from build123d import *

# Parameters (mm, degrees)
SKETCH1_R           = 19
BOSS_EXTRUDE1_DEPTH = 57
SKETCH3_W           = 38
SKETCH3_H           = 38
BOSS_EXTRUDE3_DEPTH = 48
SKETCH4_R           = 6.5
BOSS_EXTRUDE4_DEPTH = 26
SKETCH5_R           = 1.5
BOSS_EXTRUDE5_DEPTH = 13
FILLET1_R           = 5
SKETCH6_R           = 2
CUT_EXTRUDE1_DEPTH  = 10
CUT_EXTRUDE2_START  = -10
SKETCH7_R           = 2
CUT_EXTRUDE2_DEPTH  = 10


with BuildPart() as part:
    # Sketch1 → Boss-Extrude1 (new body)
    with BuildSketch(Plane.XY):
        with Locations(Location((0, 0, 0), (0, 0, 180))):
            Circle(SKETCH1_R)
    extrude(amount=BOSS_EXTRUDE1_DEPTH)

    # Sketch3 → Boss-Extrude3 (add)
    with BuildSketch(Plane(origin=(0, 0, 0), x_dir=(-1, 0, 0), z_dir=(0, 0, -1))):
        Rectangle(SKETCH3_W, SKETCH3_H)
    extrude(amount=BOSS_EXTRUDE3_DEPTH)

    # Sketch4 → Boss-Extrude4 (add)
    with BuildSketch(Plane(origin=(0, 0, -48), x_dir=(-1, 0, 0), z_dir=(0, 0, -1))):
        with Locations(Location((0, 0, 0), (0, 0, 180))):
            Circle(SKETCH4_R)
    extrude(amount=BOSS_EXTRUDE4_DEPTH)

    # Sketch5 → Boss-Extrude5 (add)
    with BuildSketch(Plane.XY.offset(57)):
        with Locations(Location((0, 0, 0), (0, 0, 180))):
            Circle(SKETCH5_R)
    extrude(amount=BOSS_EXTRUDE5_DEPTH)

    # Fillet1
    fillet1_edges = [part.edges().sort_by_distance(p)[0] for p in [
        (-19, -19, -24),
        (-19, 19, -24),
        (19, 19, -24),
        (19, -19, -24),
    ]]
    fillet(fillet1_edges, radius=FILLET1_R)

    # Sketch6 → Cut-Extrude1 (cut)
    with BuildSketch(Plane.ZY.offset(19)):
        with Locations((-4, 9)):
            Circle(SKETCH6_R)
        with Locations((-4, -9)):
            Circle(SKETCH6_R)
        with Locations((-41, -9)):
            Circle(SKETCH6_R)
        with Locations((-41, 9)):
            Circle(SKETCH6_R)
    extrude(amount=-CUT_EXTRUDE1_DEPTH, mode=Mode.SUBTRACT)

    # Sketch7 → Cut-Extrude2 (cut)
    with BuildSketch(Plane(origin=(19, 0, 0), x_dir=(0, 0, -1), z_dir=(1, 0, 0)).offset(CUT_EXTRUDE2_START)):
        with Locations(Location((41, 9, 0), (0, 0, 180))):
            Circle(SKETCH7_R)
        with Locations(Location((41, -9, 0), (0, 0, 180))):
            Circle(SKETCH7_R)
        with Locations(Location((4, -9, 0), (0, 0, 180))):
            Circle(SKETCH7_R)
        with Locations(Location((4, 9, 0), (0, 0, 180))):
            Circle(SKETCH7_R)
    extrude(amount=CUT_EXTRUDE2_DEPTH, mode=Mode.SUBTRACT)


solid = part.part
Can you work these out from the model? Positions are in its coordinate system, mm. A direction names the side the tool comes from. Give positions to 0.01 mm unless a question says otherwise; leave off trailing zeros. Loops run counter-clockwise (first coordinate to the right, second up) from the corner with the lowest first, then second, coordinate; pieces in that order, holes last. Notation, with made-up numbers: M 50.25,46.25 L 78.25,46.25 A14 ccw 78.25,55.25 Z; hole C 29.25,-27.5 d6. An arc over 180 degrees is marked long. One line per item, written item: value.
1) Imagine slicing it at B-B on x = -15.5. Write out the boundary of the cut face in (y, z).
Geometry check:
outline: M -18.77,-48 L 18.77,-48 L 18.77,0 L 10.99,0 L 10.99,57 L -10.99,57 L -10.99,0 L -18.77,0 Z; hole C -9,-41 d4; hole C -9,-4 d4; hole C 9,-41 d4; hole C 9,-4 d4
2) On a 3-axis mill with a long thin cutter (end or side, diameter ignored), from which of +Z, -Z, +X, -X, +Y, -Y can I reach the whole of each face in a straight line? I mean faces 1 (the face through (-14.07, -7.648, -42.474)), 2 (the face through (-1.43, -0.45, 63.41)), 3 (the face through (-5.158, 3.955, -60.818)), 4 (the face through (13.93, 7.648, -42.474)). Say none if no direction works.
Geometry check:
face 1: -X
face 2: +Z
face 3: -Z
face 4: +X
3) Imagine slicing it at C-C on y = 9. Write out the boundary of the cut face in (x, z).
Geometry check:
outline: M -19,-48 L 19,-48 L 19,-43 L 9,-43 L 9,-39 L 19,-39 L 19,-6 L 9,-6 L 9,-2 L 19,-2 L 19,0 L 16.73,0 L 16.73,57 L -16.73,57 L -16.73,0 L -19,0 L -19,-2 L -9,-2 L -9,-6 L -19,-6 L -19,-39 L -9,-39 L -9,-43 L -19,-43 Z
4) Thinking about a two-plate mould opening in Z: for faces 5 (the face through (14, 14, 0)), 6 (the face through (4.119, 18.548, 28.101)), 7 (the face through (-9, -9, -41)), which applies, +Z half, -Z half, draft (parallel to the pull), parting line (faces both ways), or undercut?
Geometry check:
face 5: +Z half
face 6: draft
face 7: undercut
5) Imagine slicing it at D-D on z = -65. Write out the boundary of the cut face in (x, y), and give its area (3 significant figures).
Geometry check:
outline: C 0,0 d13
area: 133 mm²
6) Please list where these lines run through material, in increasing order: line 1 (Y direction, x = -13.5, z = -4); line 2 (Z direction, x = 15.5, y = 9); line 3 (Y direction, x = 17.25, z = -41).
Geometry check:
line 1: y = -19 to -11, -7 to 7, 11 to 19
line 2: z = -48 to -43, -39 to -6, -2 to 57
line 3: y = -17.8 to -11, -7 to 7, 11 to 17.8
7) I'm going to push flat-ended pins straight in: pin 1 (10 mm diameter, centred on x = -7, y = 11.5, fed in from +Z); pin 2 (6 mm diameter, centred on x = 8.5, y = -7, fed in from -Z); pin 3 (8 mm diameter, centred on x = 0.5, z = -51.5, fed in from -Y); pin 4 (2.5 mm diameter, centred on y = 9, z = -41, fed in from -X). Where does each tip first touch, or does it pass through?
Geometry check:
pin 1: stops at z = 57
pin 2: stops at z = -48
pin 3: stops at y = -19
pin 4: stops at x = -9
8) Imagine slicing it at A-A on z = -41. Write out the boundary of the cut face in (x, y).
Geometry check:
outline: M -19,-14 A5 ccw -14,-19 L 14,-19 A5 ccw 19,-14 L 19,-11 L 9,-11 L 9,-7 L 19,-7 L 19,7 L 9,7 L 9,11 L 19,11 L 19,14 A5 ccw 14,19 L -14,19 A5 ccw -19,14 L -19,11 L -9,11 L -9,7 L -19,7 L -19,-7 L -9,-7 L -9,-11 L -19,-11 Z
